Solid Edge part; units mm, degrees
sketch "Sketch1" plane through (0, 0, 0) normal (0, 0, 1) x (1, 0, 0)
  line L0 (12, 16) -> (12, 0)
  line L1 (12, 0) -> (-12, 0)
  line L2 (-12, 0) -> (-12, 16)
  line L3 (12, 16) -> (-12, 16)
  dimension "D1" = 12
  dimension "D2" = 12
extrude "Protrusion1" add sketch "Sketch1" along normal blind 1
sketch "Sketch2" plane through (0, 10, 1) normal (0, 0, 1) x (1, 0, 0)
  circle A0 centre (8, 0) radius 3
  circle A1 centre (-8, 0) radius 3
  dimension "D1" = 8
  dimension "D2" = 8
extrude "Screwholes" add sketch "Sketch2" along normal blind 3
sketch "Sketch3" plane through (-7.5, 10, 4) normal (0, 0, 1) x (1, 0, 0)
  circle A0 centre (-0.5, 0) radius 2.5
  circle A1 centre (15.5, 0) radius 2.5
extrude "Cutout___Holes" cut sketch "Sketch3" against normal blind 1
hole "Hole1" at (-8, 10, 3) direction (0, 0, -1) diameter 2.6 end up to next
hole "Hole2" at (8, 10, 3) direction (0, 0, -1) diameter 2.6 end up to next
sketch "Sketch4" plane through (0, 10, 1) normal (0, 0, 1) x (1, 0, 0)
  line L0 (-8, -10) -> (-8, -9)
  line L1 (-8, -9) -> (8, -9)
  line L2 (8, -9) -> (8, -10)
  line L3 (8, -10) -> (-8, -10)
  line L4 (12, 6) -> (12, 5)
  line L5 (12, 5) -> (-12, 5)
  line L6 (-12, 5) -> (-12, 6)
  line L7 (-12, 6) -> (12, 6)
  dimension "D1" = 8
  dimension "D2" = 12
extrude "Walls" add sketch "Sketch4" along normal blind 4
sketch "Sketch5" plane through (0, 0, 2.5) normal (0, -1, 0) x (1, 0, 0)
  line L0 (2, 1.5) -> (3.57, 1.5)
  line L1 (3.57, 1.5) -> (3.57, 2.5)
  line L2 (-3.57, 2.5) -> (3.57, 2.5)
  line L3 (-3.57, 2.5) -> (-3.57, 1.5)
  line L4 (-3.57, 1.5) -> (-2, 1.5)
  arc A0 (2, 1.5) -> (-2, 1.5) centre (0, 1.5) cw
  dimension "D1" = 3.57
extrude "Cutout1" cut sketch "Sketch5" against normal through all
fillet "Round___body" radius 4 2 edges at (12, 0, 0.5) (-12, 0, 0.5)
properties material "ABS Plastic, high impact"
Can you work these out from the model? Positions are in its coordinate system, mm. A direction names the side the tool comes from. Round coordinates to 2 decimals unless told otherwise and drop trailing zeros. Write each loop counter-clockwise with the first axis right and the second up, starting at its lowest first coordinate (ties: lowest second). Pieces come first, ordered by that corner, then holes. Notation, with made-up numbers: (-8, -29.5) -> (37, -29.5) arc R16 ccw to (37, -3.5) -> close; hole circle Ø10 at (-38, 79.25). An arc over 180 degrees is marked (long way). Use one line per item in the form item = value. Start each with the question number.
Q1. Imagine slicing it at A-A (y = 10). Please give me the cut outline in (x, z), then the cut area to 3 significant figures.
Q2. We'd pull the mould along X, two halves only. Please class faces 6 (the face through (8, 0.5, 3)), 7 (the face through (-2.8, 15.5, 4)), 8 (the face through (7.8, 15.5, 5)): +X half, -X half, draft (parallel to the pull), parting line (faces both ways), or undercut.
Q3. If I drill on probe 1 along Y at (x, z) = (-2.5, 3.95); probe 2 along Y at (x, z) = (-9.5, 3.85); probe 3 along Z at (x, y) = (-5.75, 4.75), over which ranges is the centre line in solid material (lowest first)? Write a range as [from, to].
Q4. I'm going to push flat-ended pins straight in: P1, Ø2.5, axis at x = 7, y = 10.5, coming from the +Z side; P2, Ø0.5, axis at y = 0.5, z = 4.5, coming from the -X side; P3, Ø3, axis at y = 13, z = 3.5, coming from the +X side. Where does each tip first touch, or does it pass through?
Q5. Imagine slicing it at D-D (z = 4.65). Please give me the cut outline in (x, y), then the cut area to 3 significant figures.
Q6. Imagine slicing it at C-C (z = 0.45). Please give me the cut outline in (x, y).
Q7. Which directions (+Z, -Z, +X, -X, +Y, -Y) give clear straight access to the entire face, cutting with the end or side of a thin tool? Please do faces 1 (the face through (0, 16, 1)), 2 (the face through (0, 0, 1)), 3 (the face through (0, 8, 1)), 4 (the face through (-10, 12, 4)), 5 (the face through (-2.8, 0.5, 4)).
Q8. Imagine slicing it at B-B (z = 1.7). Please give me the cut outline in (x, y), then the cut area to 3 significant figures.
Worked out:
q1.outline = (-12, 0) -> (-9.3, 0) -> (-9.3, 3) -> (-10.5, 3) -> (-10.5, 4) -> (-11, 4) -> (-11, 1) -> (-12, 1) -> close; (-6.7, 0) -> (6.7, 0) -> (6.7, 3) -> (5.5, 3) -> (5.5, 4) -> (5, 4) -> (5, 1) -> (-5, 1) -> (-5, 4) -> (-5.5, 4) -> (-5.5, 3) -> (-6.7, 3) -> close; (9.3, 0) -> (12, 0) -> (12, 1) -> (11, 1) -> (11, 4) -> (10.5, 4) -> (10.5, 3) -> (9.3, 3) -> close
q1.area = 34.4 mm^2
q2.face_6 = +X half
q2.face_7 = undercut
q2.face_8 = draft
q3.probe_1 = [0, 1], [15, 16]
q3.probe_2 = [7.4, 8], [12, 12.6], [15, 16]
q3.probe_3 = [0, 1]
q4.P1 = 3
q4.P2 = -8
q4.P3 = 10.6
q5.outline = (-12, 15) -> (-3.57, 15) -> (-3.57, 16) -> (-12, 16) -> close; (-8, 0) -> (-3.57, 0) -> (-3.57, 1) -> (-8, 1) -> close; (3.57, 0) -> (8, 0) -> (8, 1) -> (3.57, 1) -> close; (3.57, 15) -> (12, 15) -> (12, 16) -> (3.57, 16) -> close
q5.area = 25.7 mm^2
q6.outline = (-12, 4) arc R4 ccw to (-8, 0) -> (8, 0) arc R4 ccw to (12, 4) -> (12, 16) -> (-12, 16) -> close; hole circle Ø2.6 at (-8, 10); hole circle Ø2.6 at (8, 10)
q7.face_1 = +Z, -Z, +X, -X, +Y
q7.face_2 = +Z, -Z, +X, -X, -Y
q7.face_3 = +Z
q7.face_4 = +Z, +X, -X
q7.face_5 = +Z, +Y, -Y
q8.outline = (-12, 15) -> (12, 15) -> (12, 16) -> (-12, 16) -> close; circle Ø6 at (-8, 10); (-8, 0) -> (8, 0) -> (8, 1) -> (-8, 1) -> close; circle Ø6 at (8, 10); hole circle Ø2.6 at (-8, 10); hole circle Ø2.6 at (8, 10)
q8.area = 85.9 mm^2
